```python
from build123d import *

# Parameters (mm, degrees)
SKETCH001_R     = 5.5499
POCKET_DEPTH    = 6.35
SKETCH002_R     = 28.575
POCKET001_DEPTH = 152.4
SKETCH003_R     = 3.81
POCKET002_DEPTH = 6.35


with BuildPart() as part:
    # Sketch → Revolution (revolve)
    with BuildSketch(Plane.XY):
        Polygon((0, 76.2), (-76.2, 76.2), (-76.2, 69.85), (-31.75, 69.85), (-31.75, 6.35), (-76.2, 6.35), (-76.2, 0), (0, 0), align=None)
    revolve(axis=Axis((0, 0, 0), (0, 1, 0)))

    # Sketch001 → Pocket (cut)
    with BuildSketch(Plane.XZ):
        with Locations((-53.1749, 0)):
            Circle(SKETCH001_R)
        with Locations((53.1749, 0)):
            Circle(SKETCH001_R)
    extrude(amount=-POCKET_DEPTH, mode=Mode.SUBTRACT)

    # Sketch002 → Pocket001 (cut)
    with BuildSketch(Plane(origin=(0, 76.2, 0), x_dir=(-1, 0, 0), z_dir=(0, 1, 0))):
        Circle(SKETCH002_R)
    extrude(amount=-POCKET001_DEPTH, mode=Mode.SUBTRACT)

    # Sketch003 → Pocket002 (cut)
    with BuildSketch(Plane(origin=(0, 76.2, 0), x_dir=(-1, 0, 0), z_dir=(0, 1, 0))):
        with Locations((-44.45, 44.45)):
            Circle(SKETCH003_R)
        with Locations((44.45, -44.45)):
            Circle(SKETCH003_R)
        with Locations((44.45, 44.45)):
            Circle(SKETCH003_R)
        with Locations((-44.45, -44.45)):
            Circle(SKETCH003_R)
    extrude(amount=-POCKET002_DEPTH, mode=Mode.SUBTRACT)


solid = part.part
```
Geometry: final body of the model. Coordinates: model frame, mm. A direction names the side the tool comes from. Round coordinates to 2 decimals unless told otherwise and drop trailing zeros. Write each loop counter-clockwise with the first axis right and the second up, starting at its lowest first coordinate (ties: lowest second). Pieces come first, ordered by that corner, then holes.
Item 1: Set-up query: faces 1 (the face through (48.256, 73.069, 44.618)), 2 (the face through (-33, 0, 1)), 3 (the face through (-58.72, 3.13, 0.24)), 4 (the face through (-33, 69.85, 1)). Return all of +Z, -Z, +X, -X, +Y, -Y with unobstructed straight access to the full face (end or side cutting, diameter ignored); none if empty.
Item 2: Section query B-B (z = -3). Return loops of the section in (x, y).
Item 3: Material intervals for L1, parallel to Y at x = -28, z = -37; L2, parallel to Z at x = -44, y = 74, sorted ascending.
Item 4: Section query C-C (x = -44.45). Return loops of the section in (y, z), plus the area to 3 significant figures.
Item 5: Pin query (flat end, axial travel): P1, Ø4.5, axis at x = -44.45, z = 44.45, coming from the +Y side; P2, Ø5, axis at y = 56.5, z = 1, coming from the +X side; P3, Ø3, axis at y = 59.5, z = -34.5, coming from the -X side; P4, Ø8, axis at x = -7.5, y = 38.5, coming from the +Z side. Return the tip coordinate at first contact, or that it passes through.
Item 6: Section query D-D (z = -63.5). Return loops of the section in (x, y).
Item 7: Mould query, pull axis Z, two halves, no side actions, for faces 5 (the face through (48.256, 73.069, -44.282)), 6 (the face through (33, 6.35, 1)), 7 (the face through (6.883, 37.656, -30.995)), 8 (the face through (47.63, 3.13, 0.24)). Classes: +Z half, -Z half, draft (parallel to the pull), parting line (faces both ways), or undercut.
Item 8: Section query A-A (x = 0). Return loops of the section in (y, z) (3 decimals), plus the area to 3 significant figures.
Completed:
1. face 1: +Y
1. face 2: +Z, -Z, +X, -X, -Y
1. face 3: -Y
1. face 4: none
2. outline: (-76.14, 0) - (-57.84, 0) - (-57.84, 6.35) - (-76.14, 6.35) - close; (-76.14, 69.85) - (-31.61, 69.85) - (-31.61, 6.35) - (-48.51, 6.35) - (-48.51, 0) - (-28.42, 0) - (-28.42, 76.2) - (-76.14, 76.2) - close; (28.42, 0) - (48.51, 0) - (48.51, 6.35) - (31.61, 6.35) - (31.61, 69.85) - (76.14, 69.85) - (76.14, 76.2) - (28.42, 76.2) - close; (57.84, 0) - (76.14, 0) - (76.14, 6.35) - (57.84, 6.35) - close
3. L1: y = 0 to 6.35, 69.85 to 76.2
3. L2: z = -62.21 to -48.23, -40.67 to 40.67, 48.23 to 62.21
4. outline: (0, -61.89) - (6.35, -61.89) - (6.35, 61.89) - (0, 61.89) - close; (69.85, -61.89) - (76.2, -61.89) - (76.2, -48.26) - (69.85, -48.26) - close; (69.85, -40.64) - (76.2, -40.64) - (76.2, 40.64) - (69.85, 40.64) - close; (69.85, 48.26) - (76.2, 48.26) - (76.2, 61.89) - (69.85, 61.89) - close
4. area: 1,480 mm2
5. P1: stops at y = 6.35
5. P2: stops at x = 31.75
5. P3: passes through
5. P4: stops at z = 31.56
6. outline: (-42.12, 0) - (42.12, 0) - (42.12, 6.35) - (-42.12, 6.35) - close; (-42.12, 69.85) - (42.12, 69.85) - (42.12, 76.2) - (-42.12, 76.2) - close
7. face 5: undercut
7. face 6: draft
7. face 7: parting line
7. face 8: undercut
8. outline: (0, -76.2) - (6.35, -76.2) - (6.35, -31.75) - (69.85, -31.75) - (69.85, -76.2) - (76.2, -76.2) - (76.2, -28.575) - (0, -28.575) - close; (0, 28.575) - (76.2, 28.575) - (76.2, 76.2) - (69.85, 76.2) - (69.85, 31.75) - (6.35, 31.75) - (6.35, 76.2) - (0, 76.2) - close
8. area: 1,610 mm2
